```python
from build123d import *

# Parameters (mm, degrees)
SKETCH_1_W         = 10
SKETCH_1_H         = 10
EXTRUDE_1_DEPTH    = 11.4
HOLE_WIZARD_M4_1_D = 3.3


with BuildPart() as part:
    # 草图1 → 凸台-拉伸1 (new body)
    with BuildSketch(Plane.XY):
        with Locations((5, 5)):
            Rectangle(SKETCH_1_W, SKETCH_1_H)
    extrude(amount=EXTRUDE_1_DEPTH)

    # M4 螺纹孔1 (through all)
    with Locations(Plane.XY.offset(11.4)):
        with Locations((5, 5)):
            Hole(HOLE_WIZARD_M4_1_D / 2)


solid = part.part
```
Source: CAD feature listing. Evaluate the final solid. Frame: model axes, mm. Round coordinates to 2 decimals unless told otherwise and drop trailing zeros. Loops run counter-clockwise (first coordinate to the right, second up) from the corner with the lowest first, then second, coordinate; pieces in that order, holes last. Notation, with made-up numbers: (58.5, 58.25) - (115.5, 58.25) arc R7 cw to (115.5, 62.25) - close; hole circle Ø8 at (15.25, -30.5). An arc over 180 degrees is marked (long way). Use CSV: the item, a comma, the result in double quotes.
Q1. Ray query, line 1 along Y through (x, z) = (5, 4); line 2 along Y through (x, z) = (6.25, 9.75). Return the intervals inside material, ascending.
Reported:
line 1,"0 to 3.35, 6.65 to 10"
line 2,"0 to 3.92, 6.08 to 10"
Q2. Mould query, pull axis Y, two halves, no side actions, for faces 1 (the cylindrical face through (6.31, 4, 5.62)), 2 (the flat face through (5, 0, 6)), 3 (the flat face through (5, 10, 6)), 4 (the flat face through (0, 5, 6)). Classes: pulls with the +Y half, pulls with the -Y half, needs draft (parallel to the pull), parting line crosses it, or undercut.
Reported:
face 1,"undercut"
face 2,"pulls with the -Y half"
face 3,"pulls with the +Y half"
face 4,"needs draft"
Q3. Section query A-A, the plane x = 5. Output: boundary loops of the cut face in (y, z), then the cut area to 3 significant figures.
Reported:
outline,"(0, 0) - (3.35, 0) - (3.35, 11.4) - (0, 11.4) - close; (6.65, 0) - (10, 0) - (10, 11.4) - (6.65, 11.4) - close"
area,"76.4 mm^2"
Q4. Section query C-C, the plane z = 6. Output: boundary loops of the cut face in (x, y).
Reported:
outline,"(0, 0) - (10, 0) - (10, 10) - (0, 10) - close; hole circle Ø3.3 at (5, 5)"
